```python
from build123d import *

# Parameters (mm, degrees)
SKETCH1_W           = 60
SKETCH1_H           = 60
BOSS_EXTRUDE1_DEPTH = 6
SKETCH2_W           = 10
SKETCH2_H           = 6
BOSS_EXTRUDE2_DEPTH = 14
BOSS_EXTRUDE3_DEPTH = 10
SKETCH4_R           = 3.625
CUT_EXTRUDE1_DEPTH  = 15
LPATTERN2_COUNT     = 3
LPATTERN2_PITCH     = 25
SKETCH5_R           = 1.625
CUT_EXTRUDE2_DEPTH  = 15
CIRPATTERN2_COUNT   = 6
FILLET1_R           = 20


with BuildPart() as part:
    # Sketch1 → Boss-Extrude1 (new body)
    with BuildSketch(Plane.XY):
        Rectangle(SKETCH1_W, SKETCH1_H)
    extrude(amount=BOSS_EXTRUDE1_DEPTH)

    # Sketch2 → Boss-Extrude2 (add)
    with BuildSketch(Plane.XY.offset(6)):
        with Locations((25, -27)):
            Rectangle(SKETCH2_W, SKETCH2_H)
    boss_extrude2 = extrude(amount=BOSS_EXTRUDE2_DEPTH)

    # Sketch3 → Boss-Extrude3 (add)
    with BuildSketch(Plane(origin=(30, 0, 0), x_dir=(0, 0, -1), z_dir=(1, 0, 0))):
        Polygon((-6, -18), (-9, -24), (-6, -24), align=None)
    boss_extrude3 = extrude(amount=-BOSS_EXTRUDE3_DEPTH)

    # Sketch4 → Cut-Extrude1 (cut)
    with BuildSketch(Plane(origin=(0, -24, 0), x_dir=(1, 0, 0), z_dir=(0, 1, 0))):
        with Locations((25, -15)):
            Circle(SKETCH4_R)
    cut_extrude1 = extrude(amount=-CUT_EXTRUDE1_DEPTH, mode=Mode.SUBTRACT)

    # LPattern2: Boss-Extrude2, Boss-Extrude3, Cut-Extrude1 ×3
    with Locations(*[(-i * LPATTERN2_PITCH, 0, 0) for i in range(1, LPATTERN2_COUNT)]):
        add(boss_extrude2)
        add(boss_extrude3)
        add(cut_extrude1, mode=Mode.SUBTRACT)

    # Sketch5 → Cut-Extrude2 (cut)
    with BuildSketch(Plane(origin=(0, 0, 0), x_dir=(-1, 0, 0), z_dir=(0, 0, -1))):
        with Locations((3.406977246, 23.321928114)):
            Circle(SKETCH5_R)
        with Locations((-3.406977246, 23.321928114)):
            Circle(SKETCH5_R)
    cut_extrude2 = extrude(amount=-CUT_EXTRUDE2_DEPTH, mode=Mode.SUBTRACT)

    # CirPattern2: Cut-Extrude2 ×6 about axis
    cirpattern2_axis = Axis((0, 4, 0), (0, 0, 1))
    for i in range(1, CIRPATTERN2_COUNT):
        add(cut_extrude2.rotate(cirpattern2_axis, i * 360 / CIRPATTERN2_COUNT), mode=Mode.SUBTRACT)

    # Fillet1
    fillet1_edges = [part.edges().sort_by_distance(p)[0] for p in [
        (-30, 30, 3),
        (30, 30, 3),
    ]]
    fillet(fillet1_edges, radius=FILLET1_R)


solid = part.part
```
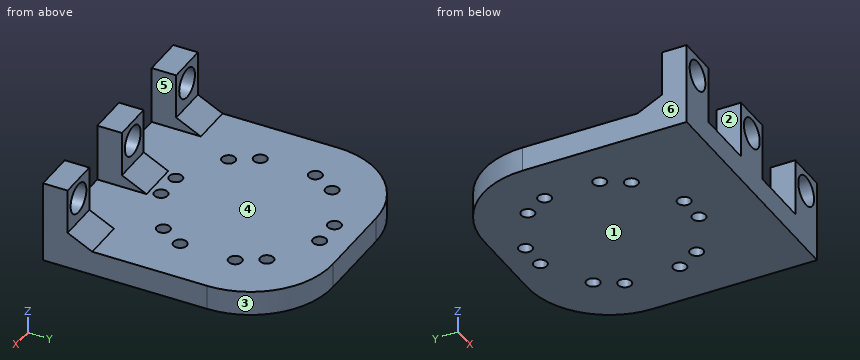
Work out the finished part from the listing and answer in its coordinate system (mm). Face numbers are marked on the shaded views. A direction names the side the tool comes from. Round coordinates to 2 decimals unless told otherwise and drop trailing zeros. Write each loop counter-clockwise with the first axis right and the second up, starting at its lowest first coordinate (ties: lowest second). Pieces come first, ordered by that corner, then holes.
1) Determine the mould class of the marked faces 1, 2 and 3 for opening direction X: pulls with the +X half, pulls with the -X half, needs draft (parallel to the pull), parting line crosses it, or undercut.
2) Flat-ended cylindrical pins translate along their axes: P1, Ø5, axis at x = 15.03, y = 16.61, coming from the +Z side; P2, Ø6, axis at y = 21, z = 4, coming from the +X side; P3, Ø5, axis at x = -24, z = 17, coming from the +Y side. Find the tip coordinate at first contact, or state that the pin passes through.
3) Consider probe 1 along X at (y, z) = (-26.5, 15) (3 decimals); probe 2 along X at (y, z) = (-27, 7.5); probe 3 along Y at (x, z) = (-16, 5.75). Determine where each line is inside the solid, lowest interval first.
4) A cutting plane is placed at C-C on z = 15. Determine the outline of the cut face in (x, y) (3 decimals), and give its area (3 significant figures).
5) A cutting plane is placed at B-B on x = 0. Determine the outline of the cut face in (y, z) (3 decimals), and give its area (4 significant figures).
6) A cutting plane is placed at A-A on z = 8.25. Determine the outline of the cut face in (x, y).
7) A cutting plane is placed at D-D on x = 23. Determine the outline of the cut face in (y, z).
8) Which of the six approach directions +Z, -Z, +X, -X, +Y, -Y give full straight-line access (tool end or side, diameter ignored) to the marked faces 4, 5 and 6?
Entries:
1. face 1: needs draft
1. face 2: undercut
1. face 3: pulls with the +X half
2. P1: stops at z = 6
2. P2: stops at x = 28.33
2. P3: stops at y = -24
3. probe 1: x = -30 to -28.625, -21.375 to -20, -5 to -3.625, 3.625 to 5, 20 to 21.375, 28.625 to 30
3. probe 2: x = -30 to -20, -5 to 5, 20 to 30
3. probe 3: y = -30 to -9.92, -7.31 to 15.31, 17.92 to 29.08
4. outline: (-30, -30) - (-28.625, -30) - (-28.625, -24) - (-30, -24) - close; (-21.375, -30) - (-20, -30) - (-20, -24) - (-21.375, -24) - close; (-5, -30) - (-3.625, -30) - (-3.625, -24) - (-5, -24) - close; (3.625, -30) - (5, -30) - (5, -24) - (3.625, -24) - close; (20, -30) - (21.375, -30) - (21.375, -24) - (20, -24) - close; (28.625, -30) - (30, -30) - (30, -24) - (28.625, -24) - close
4. area: 49.5 mm2
5. outline: (-30, 0) - (30, 0) - (30, 6) - (-18, 6) - (-24, 9) - (-24, 11.375) - (-30, 11.375) - close; (-30, 18.625) - (-24, 18.625) - (-24, 20) - (-30, 20) - close
5. area: 409.5 mm2
6. outline: (-30, -30) - (-20, -30) - (-20, -22.5) - (-30, -22.5) - close; (-5, -30) - (5, -30) - (5, -22.5) - (-5, -22.5) - close; (20, -30) - (30, -30) - (30, -22.5) - (20, -22.5) - close
7. outline: (-30, 0) - (25.2, 0) - (25.2, 6) - (-18, 6) - (-24, 9) - (-24, 11.98) - (-30, 11.98) - close; (-30, 18.02) - (-24, 18.02) - (-24, 20) - (-30, 20) - close
8. face 4: +Z, +Y
8. face 5: +Z, +Y, -Y
8. face 6: +Z, -Z, -X, +Y, -Y
